```python
from build123d import *

# Parameters (mm, degrees)
ESQUISSE1_R             = 3
BOSS_EXTRU_1_DEPTH      = 3
ESQUISSE2_R             = 2
BOSS_EXTRU_2_DEPTH      = 12
ESQUISSE3_R             = 1.65
ENL_V_MAT_EXTRU_1_DEPTH = 2
CHANFREIN1_SIZE         = 0.2


with BuildPart() as part:
    # Esquisse1 → Boss.-Extru.1 (new body)
    with BuildSketch(Plane(origin=(0, 0, 0), x_dir=(1, 0, 0), z_dir=(0, 1, 0))):
        with Locations(Location((0, 0, 0), (0, 0, 270))):
            Circle(ESQUISSE1_R)
    extrude(amount=BOSS_EXTRU_1_DEPTH)

    # Esquisse2 → Boss.-Extru.2 (add)
    with BuildSketch(Plane(origin=(0, 3, 0), x_dir=(1, 0, 0), z_dir=(0, 1, 0))):
        with Locations(Location((0, 0, 0), (0, 0, 270))):
            Circle(ESQUISSE2_R)
    extrude(amount=BOSS_EXTRU_2_DEPTH)

    # Esquisse3 → Enlèv. mat.-Extru.1 (cut)
    with BuildSketch(Plane.XZ):
        with Locations(Location((0, 0, 0), (0, 0, 270))):
            Circle(ESQUISSE3_R)
    extrude(amount=-ENL_V_MAT_EXTRU_1_DEPTH, mode=Mode.SUBTRACT)

    # Chanfrein1
    chanfrein1_edges = [part.edges().sort_by_distance(p)[0] for p in [
        (0, 0, 1.65),
        (0, 0, -3),
        (0, 3, -3),
        (0, 3, -2),
        (0, 15, -2),
    ]]
    chamfer(chanfrein1_edges, length=CHANFREIN1_SIZE)


solid = part.part
```
Check sheet for the modelled part. Datum: model origin and axes. Units: mm. A direction names the side the tool comes from. Round coordinates to 2 decimals unless told otherwise and drop trailing zeros. Order: outer loops, then holes, each group sorted by start corner. A loop starts at its lowest first (then second) coordinate and runs counter-clockwise, first axis right, second up. Notation, with made-up numbers: (17, 62.25) -> (68, 62.25) arc R15 cw to (68, 91.25) -> close; hole circle Ø7 at (14, -40). An arc over 180 degrees is marked (long way). One line per item, written item: value. Start each with the question number.
Q1. Cross-section at B-B (x = 0). Record the boundary of the cut face in (y, z), and give its area (3 significant figures).
Q2. Cross-section at D-D (y = 3.5). Record the boundary of the cut face in (x, z), and give its area (3 significant figures).
Q3. Set-up check for faces 1 (the face through (0.9, 1.48, 2.86)), 2 (the face through (-1, 1.09, 1.31)): record each of +Z, -Z, +X, -X, +Y, -Y from which the full face is reachable in a straight line by a thin tool's end or side.
Q4. Cross-section at A-A (z = 0). Record the boundary of the cut face in (x, y).
Q5. Thickness scan on line 1 (X direction, y = 1.5, z = 0); line 2 (Y direction, x = -0.2, z = -2.25); line 3 (Y direction, x = -0.1, z = -0.6). Record the ranges inside material, lowest first.
Q6. Cross-section at C-C (y = 1.5). Record the boundary of the cut face in (x, z), and give its area (3 significant figures).
Q7. Mould release check, pull along X, two halves, no side actions. Record for faces 3 (the face through (0, 2, 0)), 4 (the face through (0, 15, 0)), 5 (the face through (-2, 9, 0)): pulls with the +X half, pulls with the -X half, needs draft (parallel to the pull), parting line crosses it, or undercut.
Q8. Gauge pin test, flat ends, axial feed: pin 1 Ø1.5 at (x, z) = (-2, -2) entering from +Y; pin 2 Ø1.5 at (y, z) = (8.5, 1.5) entering from +X; pin 3 Ø1 at (x, y) = (0.5, 6.5) entering from +Z. Record the tip position at first contact, or that the pin passes through.
Completed:
1. outline: (0, -2.8) -> (0.2, -3) -> (2.8, -3) -> (3, -2.8) -> (3, -2.2) -> (3.2, -2) -> (14.8, -2) -> (15, -1.8) -> (15, 1.8) -> (14.8, 2) -> (3.2, 2) -> (3, 2.2) -> (3, 2.8) -> (2.8, 3) -> (0.2, 3) -> (0, 2.8) -> (0, 1.85) -> (0.2, 1.65) -> (2, 1.65) -> (2, -1.65) -> (0.2, -1.65) -> (0, -1.85) -> close
1. area: 59.3 mm²
2. outline: circle Ø4 at (0, 0)
2. area: 12.6 mm²
3. face 1: +Y, -Y
3. face 2: -Y
4. outline: (-3, 0.2) -> (-2.8, 0) -> (-1.85, 0) -> (-1.65, 0.2) -> (-1.65, 2) -> (1.65, 2) -> (1.65, 0.2) -> (1.85, 0) -> (2.8, 0) -> (3, 0.2) -> (3, 2.8) -> (2.8, 3) -> (2.2, 3) -> (2, 3.2) -> (2, 14.8) -> (1.8, 15) -> (-1.8, 15) -> (-2, 14.8) -> (-2, 3.2) -> (-2.2, 3) -> (-2.8, 3) -> (-3, 2.8) -> close
5. line 1: x = -3 to -1.65, 1.65 to 3
5. line 2: y = 0 to 3
5. line 3: y = 2 to 15
6. outline: circle Ø6 at (0, 0); hole circle Ø3.3 at (0, 0)
6. area: 19.7 mm²
7. face 3: undercut
7. face 4: needs draft
7. face 5: parting line crosses it
8. pin 1: stops at y = 3.12
8. pin 2: stops at x = 1.85
8. pin 3: stops at z = 2
